```python
from build123d import *

# Parameters (mm, degrees)
SKETCH4_W                  = 106
SKETCH4_H                  = 30
BOSS_EXTRUDE2_DEPTH        = 13
SKETCH25_W                 = 106
SKETCH25_H                 = 8.6
CUT_EXTRUDE3_DEPTH         = 1
CUT_EXTRUDE3_DEPTH_BACK    = 8.3
M4X0_7_TAPPED_HOLE1_D      = 3.3
SKETCH28_W                 = 106
SKETCH28_H                 = 4.5
BOSS_EXTRUDE3_DEPTH        = 41.5
SKETCH32_W                 = 41.5
SKETCH32_H                 = 4.5
BOSS_EXTRUDE10_DEPTH       = 5
SKETCH33_W                 = 13
SKETCH33_H                 = 17.121445937
BOSS_EXTRUDE12_DEPTH       = 5
SKETCH34_W                 = 4.498886861
SKETCH34_H                 = 12.621445937
BOSS_EXTRUDE13_DEPTH       = 7
SKETCH35_W                 = 54.5
SKETCH35_H                 = 4.5
BOSS_EXTRUDE14_DEPTH       = 40
SKETCH36_W                 = 5
SKETCH36_H                 = 20
BOSS_EXTRUDE15_DEPTH       = 13.12
F_8_0_199_DIAMETER_HOLE1_D = 5.0546
SKETCH39_R                 = 7
CUT_EXTRUDE4_DEPTH         = 10
M2_CLEARANCE_HOLE1_D       = 2.4
SKETCH43_W                 = 35.304815243
SKETCH43_H                 = 4
BOSS_EXTRUDE16_DEPTH       = 70
SKETCH44_W                 = 107.027081708
SKETCH44_H                 = 13.5
BOSS_EXTRUDE17_DEPTH       = 25.5
SKETCH47_W                 = 107.027081708
SKETCH47_H                 = 8.6
CUT_EXTRUDE5_DEPTH         = 8.3
M4X0_7_TAPPED_HOLE2_D      = 3.3


with BuildPart() as part:
    # Sketch4 → Boss-Extrude2 (new body)
    with BuildSketch(Plane.XY):
        with Locations((-36.891047602, -35.322762913)):
            Rectangle(SKETCH4_W, SKETCH4_H)
    extrude(amount=-BOSS_EXTRUDE2_DEPTH)

    # Sketch25 → Cut-Extrude3 (cut, two sides)
    with BuildSketch(Plane.XY) as cut_extrude3_sk:
        with Locations((-36.891047602, -28.901316976)):
            Rectangle(SKETCH25_W, SKETCH25_H)
    extrude(amount=CUT_EXTRUDE3_DEPTH, mode=Mode.SUBTRACT)
    extrude(cut_extrude3_sk.sketch, amount=-CUT_EXTRUDE3_DEPTH_BACK, mode=Mode.SUBTRACT)

    # M4x0.7 Tapped Hole1 (through all)
    with Locations(Plane(origin=(-74.390985602, -20.322762913, -4.15), x_dir=(0, 0, 1), z_dir=(0, 1, 0))):
        with Locations((0, 0), (0, 25), (-0.055677319, 74.999938), (0, 50)):
            Hole(M4X0_7_TAPPED_HOLE1_D / 2)

    # Sketch28 → Boss-Extrude3 (add)
    with BuildSketch(Plane.XY):
        with Locations((-36.891047602, -48.072762913)):
            Rectangle(SKETCH28_W, SKETCH28_H)
    extrude(amount=BOSS_EXTRUDE3_DEPTH)

    # Sketch32 → Boss-Extrude10 (add)
    with BuildSketch(Plane.ZY.offset(89.891047602)):
        with Locations((20.75, -48.072762913)):
            Rectangle(SKETCH32_W, SKETCH32_H)
    extrude(amount=BOSS_EXTRUDE10_DEPTH)

    # Sketch33 → Boss-Extrude12 (add)
    with BuildSketch(Plane.ZY.offset(89.891047602)):
        with Locations((-6.5, -41.762039945)):
            Rectangle(SKETCH33_W, SKETCH33_H)
    extrude(amount=BOSS_EXTRUDE12_DEPTH)

    # Sketch34 → Boss-Extrude13 (add)
    with BuildSketch(Plane.XY):
        with Locations((-92.641604172, -39.512039945)):
            Rectangle(SKETCH34_W, SKETCH34_H)
    extrude(amount=BOSS_EXTRUDE13_DEPTH)

    # Sketch35 → Boss-Extrude14 (add)
    with BuildSketch(Plane.ZY.offset(94.891047602)):
        with Locations((14.25, -48.072762913)):
            Rectangle(SKETCH35_W, SKETCH35_H)
    extrude(amount=BOSS_EXTRUDE14_DEPTH)

    # Sketch36 → Boss-Extrude15 (add)
    with BuildSketch(Plane(origin=(0, -45.822762913, 0), x_dir=(1, 0, 0), z_dir=(0, 1, 0))):
        with Locations((-93.41812931, -31.5)):
            Rectangle(SKETCH36_W, SKETCH36_H)
    extrude(amount=BOSS_EXTRUDE15_DEPTH)

    # #8 (0.199) Diameter Hole1 (through all)
    with Locations(Plane(origin=(-80.669073904, -45.822762913, 14.25), x_dir=(0, 0, 1), z_dir=(0, 1, 0))):
        with Locations((0, 0), (0, 91.778026302), (0, 81.778026302), (0, 10)):
            Hole(F_8_0_199_DIAMETER_HOLE1_D / 2)

    # Sketch39 → Cut-Extrude4 (cut)
    with BuildSketch(Plane(origin=(0, -45.822762913, 0), x_dir=(1, 0, 0), z_dir=(0, 1, 0))):
        with Locations((-115.41812931, -14.25)):
            Circle(SKETCH39_R)
    extrude(amount=-CUT_EXTRUDE4_DEPTH, mode=Mode.SUBTRACT)

    # M2 Clearance Hole1 (through all)
    with Locations(Plane(origin=(-107.41812931, -45.822762913, 14.25), x_dir=(0, 0, 1), z_dir=(0, 1, 0))):
        with Locations((0, 0), (8.000007036, -8.002918292), (-7.999992964, -8.002918292), (0, -16)):
            Hole(M2_CLEARANCE_HOLE1_D / 2)

    # Sketch43 → Boss-Extrude16 (add)
    with BuildSketch(Plane(origin=(0, -50.322762913, 0), x_dir=(-1, 0, 0), z_dir=(0, -1, 0))):
        Polygon((95.586232359, -37.5), (95.586232359, -41.5), (134.891047602, -41.5), (134.891047602, -37.5), (130.891047602, -37.5), align=None)
        Polygon((130.891047602, -37.5), (134.891047602, -37.5), (134.891047602, 13), (130.891047602, 13), (130.891047602, 9), align=None)
        with Locations((113.238639981, 11)):
            Rectangle(SKETCH43_W, SKETCH43_H)
    extrude(amount=BOSS_EXTRUDE16_DEPTH)

    # Sketch44 → Boss-Extrude17 (add)
    with BuildSketch(Plane(origin=(0, -45.822762913, 0), x_dir=(1, 0, 0), z_dir=(0, 1, 0))):
        with Locations((-37.404588456, -34.75)):
            Rectangle(SKETCH44_W, SKETCH44_H)
    extrude(amount=BOSS_EXTRUDE17_DEPTH)

    # Sketch47 → Cut-Extrude5 (cut)
    with BuildSketch(Plane(origin=(0, 0, 28), x_dir=(-1, 0, 0), z_dir=(0, 0, -1))):
        with Locations((37.404588456, -28.902762913)):
            Rectangle(SKETCH47_W, SKETCH47_H)
    extrude(amount=-CUT_EXTRUDE5_DEPTH, mode=Mode.SUBTRACT)

    # M4x0.7 Tapped Hole2 (through all)
    with Locations(Plane(origin=(-74.391047602, -20.322762913, 32.71), x_dir=(0, 0, 1), z_dir=(0, 1, 0))):
        with Locations((0, 0), (0, 25), (0, 50), (0, 75)):
            Hole(M4X0_7_TAPPED_HOLE2_D / 2)


solid = part.part
```
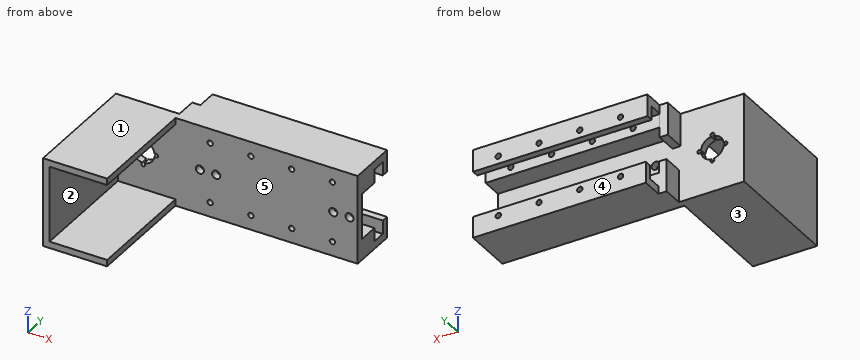
Geometry: final body of the model. Coordinates: model frame, mm. Face numbers are marked on the shaded views. A direction names the side the tool comes from. Coordinates: 2 decimals unless noted, no trailing zeros. Order: outer loops, then holes, each group sorted by start corner. A loop starts at its lowest first (then second) coordinate and runs counter-clockwise, first axis right, second up. Notation, with made-up numbers: (15, 3) - (72, 3) arc R33 cw to (72, 31) - close; hole circle Ø9 at (62.25, 79). An arc over 180 degrees is marked (long way). Write each question's results on one line, items separated by ' | '.
1) Pull-direction query (Z, two-part tool) for the marked faces 3, 4 and 5; classes: pulls with the +Z half, pulls with the -Z half, needs draft (parallel to the pull), parting line crosses it, or undercut.
Results list:
face 3: pulls with the -Z half | face 4: needs draft | face 5: undercut
2) Section C-C, the plane x = -41.5. Return loops of the section in (y, z).
Results list:
outline: (-50.32, -13) - (-20.32, -13) - (-20.32, 0) - (-24.6, 0) - (-24.6, -8.3) - (-33.2, -8.3) - (-33.2, 0) - (-45.82, 0) - (-45.82, 28) - (-33.2, 28) - (-33.2, 36.3) - (-24.6, 36.3) - (-24.6, 28) - (-20.32, 28) - (-20.32, 41.5) - (-50.32, 41.5) - close
3) Section D-D, the plane z = 26. Return loops of the section in (x, y), plus the area to 3 significant figures.
Results list:
outline: (-134.89, -120.32) - (-130.89, -120.32) - (-130.89, -50.32) - (16.11, -50.32) - (16.11, -45.82) - (-90.92, -45.82) - (-90.92, -32.7) - (-95.92, -32.7) - (-95.92, -45.82) - (-134.89, -45.82) - close | area: 1,030 mm^2
4) Section B-B, the plane y = -66. Return loops of the section in (x, z), plus the area to 3 significant figures.
Results list:
outline: (-134.89, -13) - (-95.59, -13) - (-95.59, -9) - (-130.89, -9) - (-130.89, 37.5) - (-95.59, 37.5) - (-95.59, 41.5) - (-134.89, 41.5) - close | area: 500 mm^2
5) Pin query (flat end, axial travel): pin 1 (1.5 mm diameter, centred on x = -30.5, z = 10, fed in from -Y); pin 2 (3 mm diameter, centred on x = -115.42, z = 22.25, fed in from +Y); pin 3 (4 mm diameter, centred on y = -38, z = 33.5, fed in from -X); pin 4 (3 mm diameter, centred on x = -49.39, z = 32.71, fed in from +Y). Return the tip coordinate at first contact, or that it passes through.
Results list:
pin 1: y = -50.32 | pin 2: y = -45.82 | pin 3: x = -95.92 | pin 4: through
6) Section A-A, the plane z = 32.71. State how many separate pieces and enclosed holes the cut face has, plus the area to 3 significant figures.
Results list:
separate pieces: 10 | enclosed holes: 0 | area: 2,550 mm^2
7) Set-up query: the marked faces 1 and 2. Return all of +Z, -Z, +X, -X, +Y, -Y with unobstructed straight access to the full face (end or side cutting, diameter ignored); none if empty.
Results list:
face 1: +Z, +X, -X, +Y, -Y | face 2: +X, -Y
8) Line query: line 1 (X direction, y = -37, z = 32.71); line 2 (Z direction, x = 7, y = -33); line 3 (Z direction, x = -112, y = -53.5). Output: solid intervals per line, ascending. Write a range as from..to.
Results list:
line 1: -95.92..-76.04, -72.74..-51.04, -47.74..-26.04, -22.74..-1.04, 2.26..16.11 | line 2: -13..-8.3, 36.3..41.5 | line 3: -13..-9, 37.5..41.5
